```python
from build123d import *

# Parameters (mm, degrees)
CHAMFER_1_SIZE      = 0.5
CUT_EXTRUDE_START   = -25
CUT_EXTRUDE_1_DEPTH = 25


with BuildPart() as part:
    # Sketch 1 → Revolve 1 (revolve)
    with BuildSketch(Plane.XY, mode=Mode.PRIVATE) as revolve_1_sk:
        Polygon((0, 0), (0, 8.5), (-30, 8.5), (-30, 10), (-324.998327755, 10), (-324.998327755, 9), (-328.998327755, 9), (-328.998327755, 10), (-331.998327755, 10), (-331.998327755, 8.5), (-362.998327755, 8.5), (-362.998327755, 7.75), (-364.398327755, 7.75), (-364.398327755, 8.5), (-366.498327755, 8.5), (-366.498327755, 0), align=None)
    revolve(revolve_1_sk.sketch.rotate(Axis((-850.209513438, 0, 0), (1, 0, 0)), 90), axis=Axis((-850.209513438, 0, 0), (1, 0, 0)))

    # Chamfer 1
    chamfer_1_edges = [part.edges().sort_by_distance(p)[0] for p in [
        (-324.998327755, 0, -10),
        (-30, 0, -10),
        (0, 0, -8.5),
        (-366.498327755, 0, -8.5),
    ]]
    chamfer(chamfer_1_edges, length=CHAMFER_1_SIZE)

    # Sketch 2 → Cut-Extrude 1 (cut)
    with BuildSketch(Plane(origin=(0, 0, 0), x_dir=(0, 0, -1), z_dir=(1, 0, 0)).offset(CUT_EXTRUDE_START)):
        with BuildLine():
            Line((-5.477225575, 6.5), (5.477225575, 6.5))
            ThreePointArc((5.477225575, 6.5), (0, 8.5), (-5.477225575, 6.5))
        make_face()
    extrude(amount=CUT_EXTRUDE_1_DEPTH, mode=Mode.SUBTRACT)


solid = part.part
```
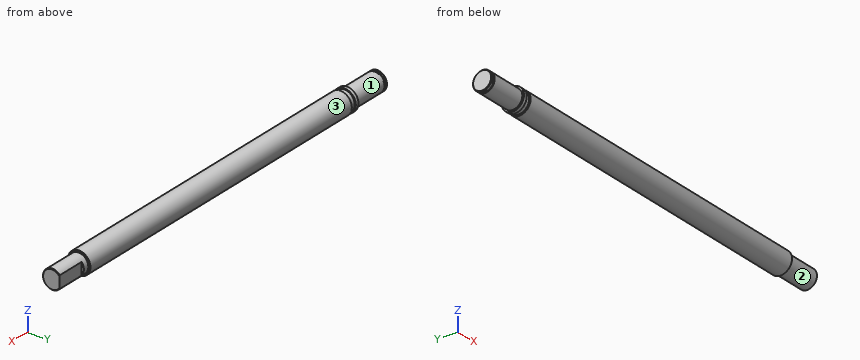
Work out the finished part from the listing and answer in its coordinate system (mm). Face numbers are marked on the shaded views. A direction names the side the tool comes from. Give positions to 0.01 mm unless a question says otherwise; leave off trailing zeros. Write each loop counter-clockwise with the first axis right and the second up, starting at its lowest first coordinate (ties: lowest second). Pieces come first, ordered by that corner, then holes.
(1) The part is cut by section A-A on x = -137. Write down the section's boundary in (y, z), plus the area to 3 significant figures.
Final values:
outline: circle Ø20 at (0, 0)
area: 314 mm2
(2) Straight lines are drawn through the part: line 1 (X direction, y = 3.25, z = -9); line 2 (Z direction, x = -29, y = -6.5); line 3 (Z direction, x = -234, y = -4.25). For each, find the intervals that lie inside material, in ascending order.
Final values:
line 1: x = -332 to -329, -324.93 to -30.07
line 2: z = -5.48 to 5.48
line 3: z = -9.05 to 9.05
(3) Which of the six approach directions +Z, -Z, +X, -X, +Y, -Y give full straight-line access (tool end or side, diameter ignored) to the marked faces 1, 2 and 3?
Final values:
face 1: -X
face 2: +X
face 3: +X, -X
(4) Flat-ended cylindrical pins translate along their axes: pin 1 Ø5.5 at (y, z) = (3, 2) entering from +X; pin 2 Ø6 at (x, y) = (-190, -4) entering from -Z; pin 3 Ø1 at (y, z) = (8, 1.5) entering from +X; pin 4 Ø2 at (x, y) = (-275, 4.5) entering from -Z. Find the tip coordinate at first contact, or state that the pin passes through.
Final values:
pin 1: stops at x = 0
pin 2: stops at z = -9.95
pin 3: stops at x = -25
pin 4: stops at z = -9.37
